Could you check a few things on this model? Use its own coordinates, in mm. Give positions to 0.01 mm unless a question says otherwise; leave off trailing zeros. Loops run counter-clockwise (first coordinate to the right, second up) from the corner with the lowest first, then second, coordinate; pieces in that order, holes last. Notation, with made-up numbers: (59, 18) - (99, 18) arc R6 cw to (99, 24) - close; hole circle Ø1 at (25, -30.5). An arc over 180 degrees is marked (long way). One line per item, written item: value. Start each with the question number.
Q1. I want a section at B-B (x = 113). Please give me the cut outline in (y, z).
Q2. I'm going to push flat-ended pins straight in: P1, Ø1, axis at y = 50, z = 1.5, coming from the +X side; P2, Ø1, axis at x = 50, y = 34.5, coming from the +Z side; P3, Ø1.1, axis at x = 100.5, z = 2.5, coming from the -Y side; P4, Ø3, axis at x = 124.5, y = 34.5, coming from the +Z side. Where does each tip first touch, or does it pass through?
Q3. If I drill on line 1 (Z direction, x = 94, y = 73); line 2 (Y direction, x = 123, z = 0.5); line 3 (X direction, y = 72.5, z = 1.05), over which ranges is the centre line in solid material (lowest first)? Write a range as from..to.
Q4. I want a section at A-A (z = 2.7). Count the separate pieces of the cut face and the enclosed holes in it, then the cut area to 3 significant figures.
Q5. I want a section at D-D (x = 80). Please give me the cut outline in (y, z), then the cut area to 3 significant figures.
Q6. I want a section at C-C (y = 71). Please give me the cut outline in (x, z).
```python
from build123d import *

# Parameters (mm, degrees)
BOSS_EXTRUDE1_DEPTH = 2
SKETCH2_R           = 3
SKETCH2_R_2         = 1.75
BOSS_EXTRUDE2_DEPTH = 1.3744
FILLET1_R           = 2
CUT_EXTRUDE1_REACH  = 154.581
SKETCH3_R           = 0.8
SKETCH6_W           = 30
SKETCH6_H           = 4
BOSS_EXTRUDE4_DEPTH = 1.3744
SKETCH7_R           = 0.7
CUT_EXTRUDE3_DEPTH  = 153.581315805
FILLET2_R           = 3


with BuildPart() as part:
    # Sketch1 → Boss-Extrude1 (new body)
    with BuildSketch(Plane.XY):
        with BuildLine():
            Line((47.808137976, 76.172186055), (63.568277585, 67.076965299))
            Line((63.568277585, 67.076965299), (63.568277585, 46.547516))
            Line((63.568277585, 46.547516), (47.808137976, 37.452295245))
            ThreePointArc((47.808137976, 37.452295245), (46.709301103, 33.354422928), (50.80717342, 32.255586055))
            Line((50.80717342, 32.255586055), (69.568277585, 43.082671869))
            Line((69.568277585, 43.082671869), (69.568277585, 55.255795635))
            Line((69.568277585, 55.255795635), (102.168277585, 55.255795635))
            Line((102.168277585, 55.255795635), (102.168277585, 44.800797075))
            Line((102.168277585, 44.800797075), (123.906537976, 32.255586055))
            ThreePointArc((123.906537976, 32.255586055), (128.004410293, 33.354422928), (126.90557342, 37.452295245))
            Line((126.90557342, 37.452295245), (108.905229152, 47.84034439))
            Line((108.905229152, 47.84034439), (108.905229152, 65.784136909))
            Line((108.905229152, 65.784136909), (126.90557342, 76.172186055))
            ThreePointArc((126.90557342, 76.172186055), (128.004410293, 80.270058372), (123.906537976, 81.368895245))
            Line((123.906537976, 81.368895245), (108.905229152, 72.711597862))
            Line((108.905229152, 72.711597862), (108.905229152, 82.35020472))
            Line((108.905229152, 82.35020472), (78.905229152, 82.35020472))
            Line((78.905229152, 82.35020472), (78.905229152, 65.153428503))
            Line((78.905229152, 65.153428503), (50.80717342, 81.368895245))
            ThreePointArc((50.80717342, 81.368895245), (46.709301103, 80.270058372), (47.808137976, 76.172186055))
        make_face()
    extrude(amount=BOSS_EXTRUDE1_DEPTH)

    # Sketch2 → Boss-Extrude2 (add)
    # profile 1 of 4: a face of its own
    with BuildSketch(Plane.XY.offset(2)):
        with Locations(Location((49.307655698, 78.77054065, 0), (0, 0, 180))):
            Circle(SKETCH2_R)
        with Locations(Location((49.307655698, 78.77054065, 0), (0, 0, 180))):
            Circle(SKETCH2_R_2, mode=Mode.SUBTRACT)
    # profile 2 of 4: a face of its own
    with BuildSketch(Plane.XY.offset(2)):
        with Locations(Location((49.307655698, 34.85394065, 0), (0, 0, 180))):
            Circle(SKETCH2_R)
        with Locations(Location((49.307655698, 34.85394065, 0), (0, 0, 180))):
            Circle(SKETCH2_R_2, mode=Mode.SUBTRACT)
    # profile 3 of 4: a face of its own
    with BuildSketch(Plane.XY.offset(2)):
        with Locations(Location((125.406055698, 34.85394065, 0), (0, 0, 180))):
            Circle(SKETCH2_R)
        with Locations(Location((125.406055698, 34.85394065, 0), (0, 0, 180))):
            Circle(SKETCH2_R_2, mode=Mode.SUBTRACT)
    # profile 4 of 4: a face of its own
    with BuildSketch(Plane.XY.offset(2)):
        with Locations(Location((125.406055698, 78.77054065, 0), (0, 0, 180))):
            Circle(SKETCH2_R)
        with Locations(Location((125.406055698, 78.77054065, 0), (0, 0, 180))):
            Circle(SKETCH2_R_2, mode=Mode.SUBTRACT)
    extrude(amount=BOSS_EXTRUDE2_DEPTH)

    # Fillet1
    fillet1_edges = [part.edges().sort_by_distance(p)[0] for p in [
        (69.568277585, 43.082671869, 1),
        (63.568277585, 46.547516, 1),
        (63.568277585, 67.076965299, 1),
        (78.905229152, 65.153428503, 1),
        (108.905229152, 72.711597862, 1),
        (108.905229152, 65.784136909, 1),
        (108.905229152, 47.84034439, 1),
        (102.168277585, 44.800797075, 1),
        (102.168277585, 55.255795635, 1),
        (69.568277585, 55.255795635, 1),
    ]]
    fillet(fillet1_edges, radius=FILLET1_R)

    # Sketch3 → Cut-Extrude1 (cut, up to next)
    with BuildSketch(Plane(origin=(0, 0, 0), x_dir=(-1, 0, 0), z_dir=(0, 0, -1)), mode=Mode.PRIVATE) as cut_extrude1_sk1:
        with Locations((-125.406055698, 78.77054065)):
            Circle(SKETCH3_R)
    cut_extrude1_tool1 = extrude(cut_extrude1_sk1.sketch, amount=-CUT_EXTRUDE1_REACH, mode=Mode.PRIVATE) & part.part
    # Sketch3 → Cut-Extrude1 (cut, up to next)
    with BuildSketch(Plane(origin=(0, 0, 0), x_dir=(-1, 0, 0), z_dir=(0, 0, -1)), mode=Mode.PRIVATE) as cut_extrude1_sk2:
        with Locations((-125.406055698, 34.85394065)):
            Circle(SKETCH3_R)
    cut_extrude1_tool2 = extrude(cut_extrude1_sk2.sketch, amount=-CUT_EXTRUDE1_REACH, mode=Mode.PRIVATE) & part.part
    # Sketch3 → Cut-Extrude1 (cut, up to next)
    with BuildSketch(Plane(origin=(0, 0, 0), x_dir=(-1, 0, 0), z_dir=(0, 0, -1)), mode=Mode.PRIVATE) as cut_extrude1_sk3:
        with Locations((-49.307655698, 34.85394065)):
            Circle(SKETCH3_R)
    cut_extrude1_tool3 = extrude(cut_extrude1_sk3.sketch, amount=-CUT_EXTRUDE1_REACH, mode=Mode.PRIVATE) & part.part
    # Sketch3 → Cut-Extrude1 (cut, up to next)
    with BuildSketch(Plane(origin=(0, 0, 0), x_dir=(-1, 0, 0), z_dir=(0, 0, -1)), mode=Mode.PRIVATE) as cut_extrude1_sk4:
        with Locations((-49.307655698, 78.77054065)):
            Circle(SKETCH3_R)
    cut_extrude1_tool4 = extrude(cut_extrude1_sk4.sketch, amount=-CUT_EXTRUDE1_REACH, mode=Mode.PRIVATE) & part.part
    add(cut_extrude1_tool1.solids().sort_by_distance((125.406056, 78.770541, 0))[0], mode=Mode.SUBTRACT)
    add(cut_extrude1_tool2.solids().sort_by_distance((125.406056, 34.853941, 0))[0], mode=Mode.SUBTRACT)
    add(cut_extrude1_tool3.solids().sort_by_distance((49.307656, 34.853941, 0))[0], mode=Mode.SUBTRACT)
    add(cut_extrude1_tool4.solids().sort_by_distance((49.307656, 78.770541, 0))[0], mode=Mode.SUBTRACT)

    # Sketch6 → Boss-Extrude4 (add)
    with BuildSketch(Plane.XY.offset(2)):
        with Locations((93.905229152, 80.35020472)):
            Rectangle(SKETCH6_W, SKETCH6_H)
    extrude(amount=BOSS_EXTRUDE4_DEPTH)

    # Sketch7 → Cut-Extrude3 (cut, through all)
    with BuildSketch(Plane(origin=(0, 0, 0), x_dir=(-1, 0, 0), z_dir=(0, 0, -1))):
        with Locations((-105.405229152, 80.39430472)):
            Circle(SKETCH7_R)
        with Locations(Location((-82.405229152, 80.39430472, 0), (0, 0, 180))):
            Circle(SKETCH7_R)
    extrude(amount=-CUT_EXTRUDE3_DEPTH, mode=Mode.SUBTRACT)

    # Fillet2
    fillet2_edges = [part.edges().sort_by_distance(p)[0] for p in [
        (78.905229152, 82.35020472, 1.6872),
        (108.905229152, 82.35020472, 1.6872),
    ]]
    fillet(fillet2_edges, radius=FILLET2_R)


solid = part.part
```
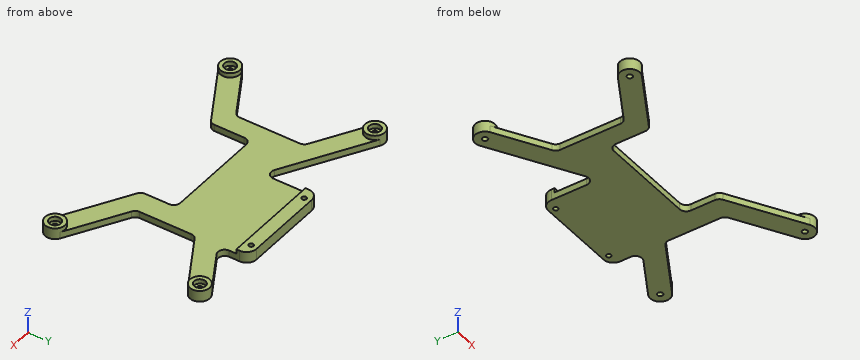
Worked answers:
1. outline: (38.55, 0) - (45.48, 0) - (45.48, 2) - (38.55, 2) - close; (68.15, 0) - (75.07, 0) - (75.07, 2) - (68.15, 2) - close
2. P1: stops at x = 108.91
2. P2: stops at z = 2
2. P3: stops at y = 55.18
2. P4: stops at z = 3.37
3. line 1: z = 0..2
3. line 2: y = 32.78..39.71, 73.92..80.85
3. line 3: x = 54.17..66.18, 78.91..120.54
4. separate pieces: 5
4. enclosed holes: 6
4. area: 188 mm²
5. outline: (55.26, 0) - (81.67, 0) - (81.67, 3.37) - (78.35, 3.37) - (78.35, 2) - (55.26, 2) - close
5. area: 57.4 mm²
6. outline: (56.77, 0) - (68.77, 0) - (68.77, 2) - (56.77, 2) - close; (78.91, 0) - (117.94, 0) - (117.94, 2) - (78.91, 2) - close
